Here's how the part is built. I have some questions about the finished solid (model axes, mm). Face numbers are marked on the shaded views. A direction names the side the tool comes from. Coordinates: 2 decimals unless noted, no trailing zeros. Write each loop counter-clockwise with the first axis right and the second up, starting at its lowest first coordinate (ties: lowest second). Pieces come first, ordered by that corner, then holes. Notation, with made-up numbers: M 55,-9 L 113,-9 A20 cw 113,4 Z; hole C -1,-13.5 d9. An arc over 180 degrees is marked long. Use a Markdown table: item, result.
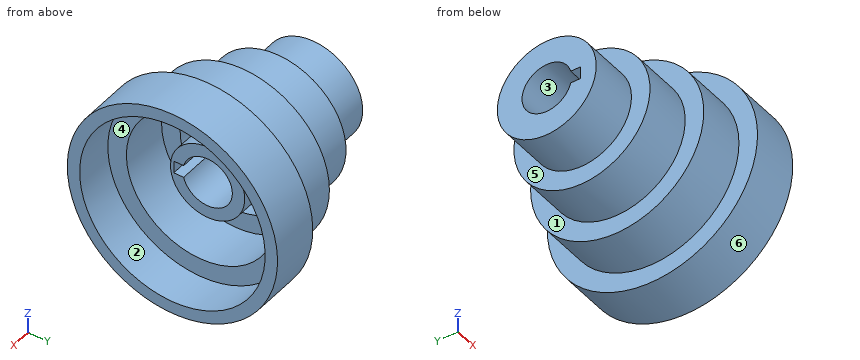
```python
from build123d import *

# Parameters (mm, degrees)
SKETCH2_R          = 20
CUT_EXTRUDE1_DEPTH = 201.124960962


with BuildPart() as part:
    # Sketch1 → Revolve1 (revolve)
    with BuildSketch(Plane.XY, mode=Mode.PRIVATE) as revolve1_sk:
        Polygon((-80, 20), (-80, 40), (-40, 40), (-40, 55), (0, 55), (0, 70), (40, 70), (40, 85), (80, 85), (80, 75), (48, 75), (48, 60), (8, 60), (8, 45), (-32, 45), (-32, 30), (40, 30), (40, 20), align=None)
    revolve(revolve1_sk.sketch.rotate(Axis((-79.321922317, 0, 0), (1, 0, 0)), 90), axis=Axis((-79.321922317, 0, 0), (1, 0, 0)))

    # Sketch2 → Cut-Extrude1 (cut, through all)
    with BuildSketch(Plane.ZY.offset(80)):
        Circle(SKETCH2_R)
        with BuildLine():
            Line((5, -19.364916731), (5, -27.364916731))
            Line((5, -27.364916731), (-5, -27.364916731))
            Line((-5, -27.364916731), (-5, -19.364916731))
            ThreePointArc((-5, -19.364916731), (0, -20), (5, -19.364916731))
        make_face()
    extrude(amount=-CUT_EXTRUDE1_DEPTH, mode=Mode.SUBTRACT)


solid = part.part
```
1. Suppose I cut it at B-B on x = -25. Write out the boundary of the cut face in (y, z), and give its area (3 significant figures).
Answers follow:
| item | result |
|---|---|
| outline | C 0,0 d110; C 0,0 d60; hole C 0,0 d90; hole M -27.36,-5 L -19.36,-5 A20 ccw long -19.36,5 L -27.36,5 Z |
| area | 4,640 mm2 |
2. I need wall thicknesses on probe 1 along Y at (x, z) = (-20, 0); probe 2 along Y at (x, z) = (61, 0); probe 3 along X at (y, z) = (-12, 52). Which ranges of each line are inside material? Lowest first, please.
Answers follow:
| item | result |
|---|---|
| probe 1 | y = -55 to -45, -30 to -27.36, 20 to 30, 45 to 55 |
| probe 2 | y = -85 to -75, 75 to 85 |
| probe 3 | x = -40 to 8 |
3. Suppose I cut it at A-A on x = 26. Write out the boundary of the cut face in (y, z), and give its area (3 significant figures).
Answers follow:
| item | result |
|---|---|
| outline | C 0,0 d140; C 0,0 d60; hole C 0,0 d120; hole M -27.36,-5 L -19.36,-5 A20 ccw long -19.36,5 L -27.36,5 Z |
| area | 5,580 mm2 |
4. Suppose I cut it at C-C on z = -57.5. Write out the boundary of the cut face in (x, y).
Answers follow:
| item | result |
|---|---|
| outline | M 0,-39.92 L 40,-39.92 L 40,-62.6 L 80,-62.6 L 80,-48.15 L 48,-48.15 L 48,-17.14 L 8,-17.14 L 8,17.14 L 48,17.14 L 48,48.15 L 80,48.15 L 80,62.6 L 40,62.6 L 40,39.92 L 0,39.92 Z |
5. Suppose I cut it at D-D on x = 52. Write out the boundary of the cut face in (y, z).
Answers follow:
| item | result |
|---|---|
| outline | C 0,0 d170; hole C 0,0 d150 |
6. Will these pins go through, and if not, where does the flat tip stop? pin 1 Ø10 at (x, y) = (-8, 8.5) entering from +Z; pin 2 Ø10 at (x, y) = (-61, -15) entering from -Z; pin 3 Ø4 at (x, y) = (-20, -24) entering from +Z.
Answers follow:
| item | result |
|---|---|
| pin 1 | stops at z = 54.89 |
| pin 2 | stops at z = -38.73 |
| pin 3 | stops at z = 50.41 |
7. We'd pull the mould along Z, two halves only. Please class the marked faces 4, 5 and 6: +Z half, -Z half, draft (parallel to the pull), parting line (faces both ways), or undercut.
Answers follow:
| item | result |
|---|---|
| face 4 | undercut |
| face 5 | draft |
| face 6 | parting line |
8. Which directions (+Z, -Z, +X, -X, +Y, -Y) give clear straight access to the entire face, cutting with the end or side of a thin tool? Please do the marked faces 1, 2 and 3.
Answers follow:
| item | result |
|---|---|
| face 1 | -X |
| face 2 | +X |
| face 3 | +X, -X |
